```python
from build123d import *

# Parameters (mm, degrees)
BOSS_EXTRUDE1_DEPTH                = 19.9898
FILLET1_R                          = 0.508
M2_5X0_45_TAPPED_HOLE1_D           = 2.05
M2_5X0_45_TAPPED_HOLE1_CSINK_D     = 2.55
M2_5X0_45_TAPPED_HOLE1_CSINK_ANGLE = 90


with BuildPart() as part:
    # Sketch1 → Boss-Extrude1 (new body)
    with BuildSketch(Plane(origin=(0, 0, 0), x_dir=(1, 0, 0), z_dir=(0, 1, 0))):
        Polygon((-2.6035, 0), (-1.30175, 2.254697139), (1.30175, 2.254697139), (2.6035, 0), (1.30175, -2.254697139), (-1.30175, -2.254697139), align=None)
    extrude(amount=BOSS_EXTRUDE1_DEPTH)

    # Fillet1
    fillet1_edges = [part.edges().sort_by_distance(p)[0] for p in [
        (-2.6035, 9.9949, 0),
        (-1.30175, 9.9949, 2.254697139),
        (1.30175, 9.9949, 2.254697139),
        (2.6035, 9.9949, 0),
        (1.30175, 9.9949, -2.254697139),
        (-1.30175, 9.9949, -2.254697139),
    ]]
    fillet(fillet1_edges, radius=FILLET1_R)

    # M2.5x0.45 Tapped Hole1 (through all)
    with Locations(Plane.ZX.offset(19.9898)):
        with Locations((0, 0)):
            CounterSinkHole(M2_5X0_45_TAPPED_HOLE1_D / 2, M2_5X0_45_TAPPED_HOLE1_CSINK_D / 2, counter_sink_angle=M2_5X0_45_TAPPED_HOLE1_CSINK_ANGLE)


solid = part.part
```
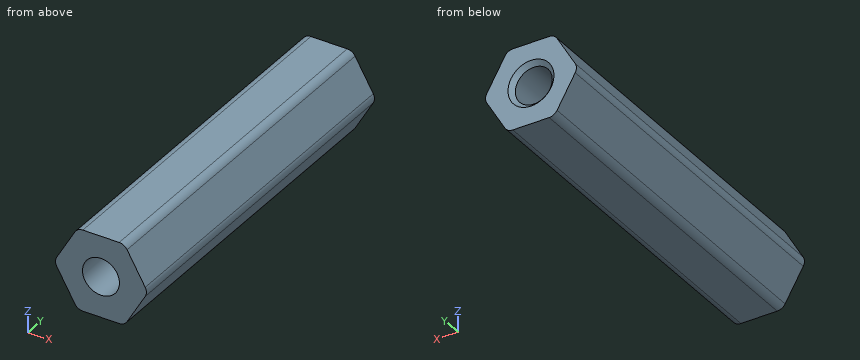
Can you work these out from the model? Positions are in its coordinate system, mm. Coordinates: 2 decimals unless noted, no trailing zeros. Loops run counter-clockwise (first coordinate to the right, second up) from the corner with the lowest first, then second, coordinate; pieces in that order, holes last. Notation, with made-up numbers: (25, 58.25) - (33, 58.25) arc R31 cw to (33, 91.25) - close; hole circle Ø8 at (52, 61). An arc over 180 degrees is marked (long way). Use a Markdown table: item, result.
Item 1: I want a section at A-A on z = 0. Please give me the cut outline in (x, y) (3 decimals).
Numbers:
| item | result |
|---|---|
| outline | (-2.525, 0) - (-1.025, 0) - (-1.025, 19.74) - (-1.275, 19.99) - (-2.525, 19.99) - close; (1.025, 0) - (2.525, 0) - (2.525, 19.99) - (1.275, 19.99) - (1.025, 19.74) - close |
Item 2: I want a section at D-D on x = -1.8. Please give me the cut outline in (y, z), and give its area (3 significant figures).
Numbers:
| item | result |
|---|---|
| outline | (0, -1.39) - (19.99, -1.39) - (19.99, 1.39) - (0, 1.39) - close |
| area | 55.6 mm2 |
Item 3: I want a section at C-C on y = 9.25. Please give me the cut outline in (x, z) (3 decimals).
Numbers:
| item | result |
|---|---|
| outline | (-2.457, -0.254) - (-1.448, -2.001) arc R0.508 ccw to (-1.008, -2.255) - (1.008, -2.255) arc R0.508 ccw to (1.448, -2.001) - (2.457, -0.254) arc R0.508 ccw to (2.457, 0.254) - (1.448, 2.001) arc R0.508 ccw to (1.008, 2.255) - (-1.008, 2.255) arc R0.508 ccw to (-1.448, 2.001) - (-2.457, 0.254) arc R0.508 ccw to start; hole circle Ø2.05 at (0, 0) |
Item 4: I want a section at B-B on x = 0. Please give me the cut outline in (y, z) (3 decimals), and give its area (3 significant figures).
Numbers:
| item | result |
|---|---|
| outline | (0, -2.255) - (19.99, -2.255) - (19.99, -1.275) - (19.74, -1.025) - (0, -1.025) - close; (0, 1.025) - (19.74, 1.025) - (19.99, 1.275) - (19.99, 2.255) - (0, 2.255) - close |
| area | 49.1 mm2 |
Item 5: Will these pins go through, and if not, where does the flat tip stop? pin 1 (2 mm diameter, centred on x = -1, z = 0, fed in from -Y); pin 2 (2.5 mm diameter, centred on x = 0, z = 0, fed in from +Y).
Numbers:
| item | result |
|---|---|
| pin 1 | stops at y = 0 |
| pin 2 | stops at y = 19.96 |
Item 6: If I drill on probe 1 along X at (y, z) = (9, 0.05); probe 2 along Z at (x, y) = (0, 6) (3 decimals); probe 3 along Z at (x, y) = (0.5, 7), over which ranges is the centre line in solid material (lowest first)? Write a range as from..to.
Numbers:
| item | result |
|---|---|
| probe 1 | x = -2.52..-1.02, 1.02..2.52 |
| probe 2 | z = -2.255..-1.025, 1.025..2.255 |
| probe 3 | z = -2.25..-0.89, 0.89..2.25 |
